Build history of the part. All positions in model axes, mm. Give positions to 0.01 mm unless a question says otherwise; leave off trailing zeros. Order: outer loops, then holes, each group sorted by start corner. A loop starts at its lowest first (then second) coordinate and runs counter-clockwise, first axis right, second up. Notation, with made-up numbers: (3, 36) - (42, 36) arc R27 cw to (42, 64) - close; hole circle Ø11 at (-36, -17.75). An arc over 180 degrees is marked (long way). One line per item, written item: value.
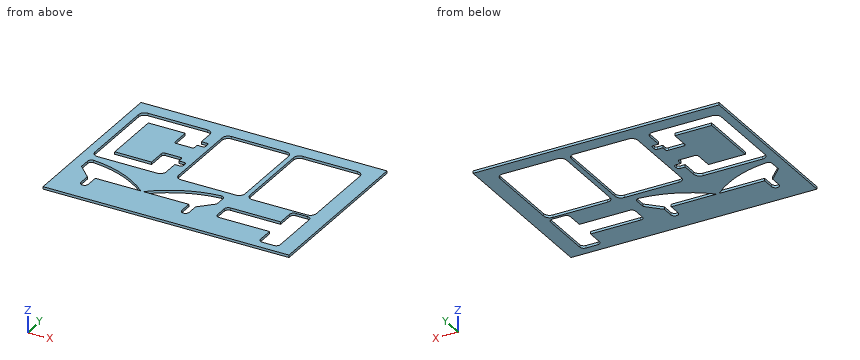
Autodesk Inventor part; units mm, degrees
ref_plane "YZ Plane" through (0, 0, 0) normal (1, 0, 0) x (0, 1, 0)
ref_plane "XZ Plane" through (0, 0, 0) normal (0, 1, 0) x (-1, 0, 0)
ref_plane "XY Plane" through (0, 0, 0) normal (0, 0, 1) x (1, 0, 0)
sketch "Sketch1" plane through (0, 0, 0) normal (0, 0, 1) x (1, 0, 0)
  arc A0 (70.6957, 42.8063) -> (77.6957, 42.8063) centre (74.1957, 42.8063) ccw
  line L0 (66.6957, 65.6673) -> (66.6957, 42.8063)
  line L1 (39.1957, 93.1673) -> (66.6957, 65.6673)
  line L2 (39.1957, 115.3063) -> (39.1957, 93.1673)
  arc A1 (46.6957, 122.8063) -> (39.1957, 115.3063) centre (46.6957, 115.3063) ccw
  arc A2 (174.1957, 67.8063) -> (46.6957, 122.8063) centre (28.9415, -93.6352) ccw
  line L3 (81.6957, 67.8063) -> (174.1957, 67.8063)
  line L4 (81.6957, 42.8063) -> (81.6957, 67.8063)
  arc A3 (66.6957, 42.8063) -> (81.6957, 42.8063) centre (74.1957, 42.8063) ccw
  circle A4 centre (299.1957, 107.8063) radius 3.5
  line L5 (275.6957, 67.8063) -> (275.6957, 42.8063)
  arc A5 (282.6957, 67.8063) -> (275.6957, 67.8063) centre (279.1957, 67.8063) ccw
  line L6 (282.6957, 42.8063) -> (282.6957, 67.8063)
  arc A6 (275.6957, 42.8063) -> (282.6957, 42.8063) centre (279.1957, 42.8063) ccw
  line L7 (286.6957, 65.6673) -> (286.6957, 42.8063)
  line L8 (314.1957, 93.1673) -> (286.6957, 65.6673)
  line L9 (314.1957, 115.3063) -> (314.1957, 93.1673)
  arc A7 (314.1957, 115.3063) -> (306.6957, 122.8063) centre (306.6957, 115.3063) ccw
  arc A8 (306.6957, 122.8063) -> (179.1957, 67.8063) centre (324.4499, -93.6352) ccw
  line L10 (271.6957, 67.8063) -> (179.1957, 67.8063)
  line L11 (271.6957, 42.8063) -> (271.6957, 67.8063)
  arc A9 (271.6957, 42.8063) -> (286.6957, 42.8063) centre (279.1957, 42.8063) ccw
  circle A10 centre (324.1957, 152.8063) radius 3.5
  circle A11 centre (219.1957, 302.8063) radius 3.5
  circle A12 centre (324.1957, 302.8063) radius 3.5
  circle A13 centre (219.1957, 152.8063) radius 3.5
  line L12 (234.1957, 177.8063) -> (234.1957, 277.8063)
  line L13 (309.1957, 177.8063) -> (234.1957, 177.8063)
  line L14 (309.1957, 277.8063) -> (309.1957, 177.8063)
  line L15 (234.1957, 277.8063) -> (309.1957, 277.8063)
  arc A14 (204.1957, 149.8063) -> (216.1957, 137.8063) centre (216.1957, 149.8063) ccw
  line L16 (204.1957, 305.8063) -> (204.1957, 149.8063)
  arc A15 (216.1957, 317.8063) -> (204.1957, 305.8063) centre (216.1957, 305.8063) ccw
  line L17 (327.1957, 317.8063) -> (216.1957, 317.8063)
  arc A16 (339.1957, 305.8063) -> (327.1957, 317.8063) centre (327.1957, 305.8063) ccw
  line L18 (339.1957, 149.8063) -> (339.1957, 305.8063)
  arc A17 (327.1957, 137.8063) -> (339.1957, 149.8063) centre (327.1957, 149.8063) ccw
  line L19 (216.1957, 137.8063) -> (327.1957, 137.8063)
  circle A18 centre (469.1957, 152.8063) radius 3.5
  circle A19 centre (364.1957, 302.8063) radius 3.5
  circle A20 centre (469.1957, 302.8063) radius 3.5
  circle A21 centre (364.1957, 152.8063) radius 3.5
  line L20 (379.1957, 177.8063) -> (379.1957, 277.8063)
  line L21 (454.1957, 177.8063) -> (379.1957, 177.8063)
  line L22 (454.1957, 277.8063) -> (454.1957, 177.8063)
  line L23 (379.1957, 277.8063) -> (454.1957, 277.8063)
  arc A22 (349.1957, 149.8063) -> (361.1957, 137.8063) centre (361.1957, 149.8063) ccw
  line L24 (349.1957, 305.8063) -> (349.1957, 149.8063)
  arc A23 (361.1957, 317.8063) -> (349.1957, 305.8063) centre (361.1957, 305.8063) ccw
  line L25 (472.1957, 317.8063) -> (361.1957, 317.8063)
  arc A24 (484.1957, 305.8063) -> (472.1957, 317.8063) centre (472.1957, 305.8063) ccw
  line L26 (484.1957, 149.8063) -> (484.1957, 305.8063)
  arc A25 (472.1957, 137.8063) -> (484.1957, 149.8063) centre (472.1957, 149.8063) ccw
  line L27 (361.1957, 137.8063) -> (472.1957, 137.8063)
  circle A26 centre (154.1957, 152.8063) radius 3.5
  circle A27 centre (49.1957, 302.8063) radius 3.5
  circle A28 centre (49.1957, 152.8063) radius 3.5
  circle A29 centre (154.1957, 302.8063) radius 3.5
  circle A30 centre (186.6957, 267.8063) radius 3.5
  circle A31 centre (186.6957, 187.8063) radius 3.5
  arc A32 (139.1957, 251.8063) -> (143.1957, 247.8063) centre (143.1957, 251.8063) ccw
  line L28 (139.1957, 287.8063) -> (139.1957, 251.8063)
  line L29 (64.1957, 287.8063) -> (139.1957, 287.8063)
  line L30 (64.1957, 167.8063) -> (64.1957, 287.8063)
  line L31 (139.1957, 167.8063) -> (64.1957, 167.8063)
  line L32 (139.1957, 203.8063) -> (139.1957, 167.8063)
  arc A33 (143.1957, 207.8063) -> (139.1957, 203.8063) centre (143.1957, 203.8063) ccw
  line L33 (175.1957, 207.8063) -> (143.1957, 207.8063)
  arc A34 (179.1957, 203.8063) -> (175.1957, 207.8063) centre (175.1957, 203.8063) ccw
  line L34 (179.1957, 195.3063) -> (179.1957, 203.8063)
  line L35 (190.1957, 195.3063) -> (179.1957, 195.3063)
  arc A35 (194.1957, 191.3063) -> (190.1957, 195.3063) centre (190.1957, 191.3063) ccw
  line L36 (194.1957, 184.3063) -> (194.1957, 191.3063)
  arc A36 (190.1957, 180.3063) -> (194.1957, 184.3063) centre (190.1957, 184.3063) ccw
  line L37 (179.1957, 180.3063) -> (190.1957, 180.3063)
  line L38 (179.1957, 149.8063) -> (179.1957, 180.3063)
  arc A37 (167.1957, 137.8063) -> (179.1957, 149.8063) centre (167.1957, 149.8063) ccw
  line L39 (46.1957, 137.8063) -> (167.1957, 137.8063)
  arc A38 (34.1957, 149.8063) -> (46.1957, 137.8063) centre (46.1957, 149.8063) ccw
  line L40 (34.1957, 305.8063) -> (34.1957, 149.8063)
  arc A39 (46.1957, 317.8063) -> (34.1957, 305.8063) centre (46.1957, 305.8063) ccw
  line L41 (167.1957, 317.8063) -> (46.1957, 317.8063)
  circle A40 centre (54.1957, 107.8063) radius 3.5
  line L42 (179.1957, 275.3063) -> (179.1957, 305.8063)
  line L43 (190.1957, 275.3063) -> (179.1957, 275.3063)
  arc A41 (194.1957, 271.3063) -> (190.1957, 275.3063) centre (190.1957, 271.3063) ccw
  line L44 (194.1957, 264.3063) -> (194.1957, 271.3063)
  arc A42 (190.1957, 260.3063) -> (194.1957, 264.3063) centre (190.1957, 264.3063) ccw
  line L45 (179.1957, 260.3063) -> (190.1957, 260.3063)
  line L46 (179.1957, 251.8063) -> (179.1957, 260.3063)
  arc A43 (175.1957, 247.8063) -> (179.1957, 251.8063) centre (175.1957, 251.8063) ccw
  line L47 (143.1957, 247.8063) -> (175.1957, 247.8063)
  circle A44 centre (341.6957, 72.8063) radius 3.5
  arc A45 (484.1957, 124.8063) -> (476.1957, 132.8063) centre (476.1957, 124.8063) ccw
  line L48 (484.1957, 20.8063) -> (484.1957, 124.8063)
  arc A46 (476.1957, 12.8063) -> (484.1957, 20.8063) centre (476.1957, 20.8063) ccw
  arc A47 (179.1957, 305.8063) -> (167.1957, 317.8063) centre (167.1957, 305.8063) ccw
  arc A48 (444.1957, 20.8063) -> (452.1957, 12.8063) centre (452.1957, 20.8063) ccw
  line L49 (444.1957, 52.8063) -> (444.1957, 20.8063)
  line L50 (342.1957, 52.8063) -> (444.1957, 52.8063)
  arc A49 (334.1957, 60.8063) -> (342.1957, 52.8063) centre (342.1957, 60.8063) ccw
  line L51 (334.1957, 84.8063) -> (334.1957, 60.8063)
  arc A50 (342.1957, 92.8063) -> (334.1957, 84.8063) centre (342.1957, 84.8063) ccw
  line L52 (444.1957, 92.8063) -> (342.1957, 92.8063)
  line L53 (444.1957, 124.8063) -> (444.1957, 92.8063)
  arc A51 (452.1957, 132.8063) -> (444.1957, 124.8063) centre (452.1957, 124.8063) ccw
  line L54 (476.1957, 132.8063) -> (452.1957, 132.8063)
  line L55 (77.6957, 67.8063) -> (77.6957, 42.8063)
  arc A52 (77.6957, 67.8063) -> (70.6957, 67.8063) centre (74.1957, 67.8063) ccw
  line L56 (70.6957, 42.8063) -> (70.6957, 67.8063)
  line L57 (452.1957, 12.8063) -> (476.1957, 12.8063)
  line L58 (17.0765, 317.8063) -> (487.0765, 317.8063) construction
  line L59 (27.0765, 327.8063) -> (27.0765, 7.8063) construction
  line L60 (17.0765, 17.8063) -> (487.0765, 17.8063) construction
  line L61 (484.1957, 7.8063) -> (484.1957, 327.8063) construction
  line L62 (516.3149, 345.8063) -> (16.3149, 345.8063)
  line L63 (16.3149, 345.8063) -> (16.3149, -4.1937)
  line L64 (16.3149, -4.1937) -> (516.3149, -4.1937)
  line L65 (516.3149, -4.1937) -> (516.3149, 345.8063)
  point P0 (179.1957, 165.0563)
  point P1 (167.0765, 67.8063)
  point P2 (172.0765, 67.8063)
  point P3 (339.1957, 305.8063)
  point P4 (27.0765, 305.8063)
  point P5 (484.1957, 20.8063)
  point P6 (452.1957, 132.8063)
  point P7 (484.1957, 124.8063)
  point P8 (342.1957, 92.8063)
  point P9 (349.1957, 149.8063)
  point P10 (349.1957, 305.8063)
  point P11 (361.1957, 137.8063)
  point P12 (216.1957, 137.8063)
  point P13 (204.1957, 149.8063)
  point P14 (46.1957, 317.8063)
  point P15 (9.1957, 345.8063)
  dimension "d20" = 30
  dimension "d21" = 30
  dimension "d22" = 30
  dimension "d23" = 40
  dimension "d24" = 4
  dimension "d25" = 4
  dimension "d26" = 4
  dimension "d27" = 4
  dimension "d28" = 7
  dimension "d29" = 7
  dimension "d30" = 7
  dimension "d31" = 7
  dimension "d32" = 75
  dimension "d33" = 12
  dimension "d34" = 12
  dimension "d35" = 12
  dimension "d36" = 12
  dimension "d37" = 120
  dimension "d38" = 40
  dimension "d39" = 25
  dimension "d40" = 15
  dimension "d41" = 15
  dimension "d42" = 15
  dimension "d43" = 15
  dimension "d44" = 15
  dimension "d49" = 140
  dimension "d50" = 5
  dimension "d51" = 50
  dimension "d52" = 145
  dimension "d53" = 12
  dimension "d54" = 123
  dimension "d55" = 145
  dimension "d57" = 12
  dimension "d61" = 500
  dimension "d62" = 350
  dimension "d64" = 30
  dimension "d65" = 28
extrude "Extrusion2" add sketch "Sketch1" along normal blind 5 contours L65 L64 L63 L62
properties part number "MarcoRompecabezas" material "MDF Medium Density Fiberboard"
(1) Slice it at D-D, the plane z = 3.65. Count the separate pieces of the cut face and the enclosed holes in it, and give its area (3 significant figures).
Completed:
separate pieces: 1
enclosed holes: 6
area: 91,500 mm²
(2) Slice it at B-B, the plane y = 280.5. Give the cut face in (x, z).
Completed:
outline: (16.31, 0) - (34.2, 0) - (34.2, 5) - (16.31, 5) - close; (64.2, 0) - (139.2, 0) - (139.2, 5) - (64.2, 5) - close; (179.2, 0) - (204.2, 0) - (204.2, 5) - (179.2, 5) - close; (339.2, 0) - (349.2, 0) - (349.2, 5) - (339.2, 5) - close; (484.2, 0) - (516.31, 0) - (516.31, 5) - (484.2, 5) - close
(3) Slice it at A-A, the plane x = 414. Give the cut face in (y, z), and give its area (3 significant figures).
Completed:
outline: (-4.19, 0) - (52.81, 0) - (52.81, 5) - (-4.19, 5) - close; (92.81, 0) - (137.81, 0) - (137.81, 5) - (92.81, 5) - close; (317.81, 0) - (345.81, 0) - (345.81, 5) - (317.81, 5) - close
area: 650 mm²
(4) Pin check, flat tip, straight feed: P1, Ø5, axis at x = 205.5, y = 145.5, coming from the -Z side. Stop position of the tip, or through.
Completed:
P1: z = 0
(5) Drill centre lines: line 1 (X direction, y = 155, z = 3.25); line 2 (X direction, y = 46.5, z = 2.4); line 3 (Y direction, x = 435.5, z = 3.8). Where is each one in solid material? Low to high.
Completed:
line 1: 16.31 to 34.2, 179.2 to 204.2, 339.2 to 349.2, 484.2 to 516.31
line 2: 16.31 to 66.7, 81.7 to 271.7, 286.7 to 444.2, 484.2 to 516.31
line 3: -4.19 to 52.81, 92.81 to 137.81, 317.81 to 345.81
(6) Slice it at C-C, the plane x = 112.5. Give the cut face in (y, z).
Completed:
outline: (-4.19, 0) - (67.81, 0) - (67.81, 5) - (-4.19, 5) - close; (106.81, 0) - (137.81, 0) - (137.81, 5) - (106.81, 5) - close; (167.81, 0) - (287.81, 0) - (287.81, 5) - (167.81, 5) - close; (317.81, 0) - (345.81, 0) - (345.81, 5) - (317.81, 5) - close
